Build history of the part. All positions in model axes, mm. Face numbers are marked on the shaded views. Coordinates: 2 decimals unless noted, no trailing zeros. Write each loop counter-clockwise with the first axis right and the second up, starting at its lowest first coordinate (ties: lowest second). Pieces come first, ordered by that corner, then holes.
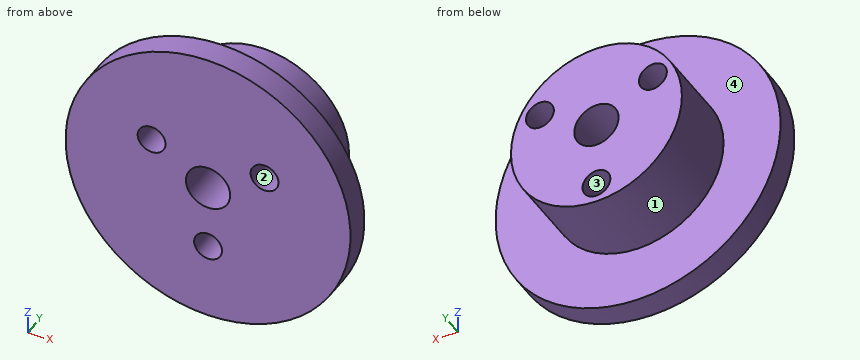
```python
from build123d import *

# Parameters (mm, degrees)
SKETCH_1_R          = 11.25
EXTRUDE_1_DEPTH     = 8
CUT_EXTRUDE_START   = -6
SKETCH_3_R          = 11.25
SKETCH_3_R_2        = 6.75
CUT_EXTRUDE_1_DEPTH = 6
SKETCH_4_R          = 1.75
SKETCH_4_R_2        = 1.1
CUT_EXTRUDE_2_DEPTH = 18.808003819


with BuildPart() as part:
    # 草图1 → 凸台-拉伸1 (new body)
    with BuildSketch(Plane(origin=(0, 0, 0), x_dir=(1, 0, 0), z_dir=(0, 1, 0))):
        with Locations(Location((0, 0, 0), (0, 0, 270))):
            Circle(SKETCH_1_R)
    extrude(amount=EXTRUDE_1_DEPTH)

    # 草图3 → 切除-拉伸1 (cut)
    with BuildSketch(Plane(origin=(0, 8, 0), x_dir=(1, 0, 0), z_dir=(0, 1, 0)).offset(CUT_EXTRUDE_START)):
        with Locations(Location((0, 0, 0), (0, 0, 270))):
            Circle(SKETCH_3_R)
        with Locations(Location((0, 0, 0), (0, 0, 270))):
            Circle(SKETCH_3_R_2, mode=Mode.SUBTRACT)
    extrude(amount=CUT_EXTRUDE_1_DEPTH, mode=Mode.SUBTRACT)

    # 草图4 → 切除-拉伸2 (cut, through all)
    with BuildSketch(Plane(origin=(0, 8, 0), x_dir=(1, 0, 0), z_dir=(0, 1, 0))):
        with Locations(Location((0, 0, 0), (0, 0, 270))):
            Circle(SKETCH_4_R)
        with Locations(Location((0, 5.15, 0), (0, 0, 270))):
            Circle(SKETCH_4_R_2)
        with Locations(Location((4.460030829, -2.575, 0), (0, 0, 270))):
            Circle(SKETCH_4_R_2)
        with Locations(Location((-4.460030829, -2.575, 0), (0, 0, 270))):
            Circle(SKETCH_4_R_2)
    extrude(amount=-CUT_EXTRUDE_2_DEPTH, mode=Mode.SUBTRACT)


solid = part.part
```
1. Saw through at D-D on y = 6.5. List the corners of the cut face in (x, z) (3 decimals).
Computed values:
outline: circle Ø13.5 at (0, 0); hole circle Ø2.2 at (-4.46, 2.575); hole circle Ø3.5 at (0, 0); hole circle Ø2.2 at (0, -5.15); hole circle Ø2.2 at (4.46, 2.575)
2. Flat gauge pins, fed straight in: pin 1 (4 mm diameter, centred on y = 2, z = -7.5, fed in from -X); pin 2 (1.5 mm diameter, centred on y = 2.5, z = -8, fed in from -X); pin 3 (1 mm diameter, centred on y = 5, z = 4, fed in from +X). Where does each tip first touch, or does it go through?
Computed values:
pin 1: stops at x = -9.81
pin 2: stops at x = -8.44
pin 3: stops at x = 5.77
3. Saw through at B-B on z = 0. List the corners of the cut face in (x, y), plus the area to 3 significant figures.
Computed values:
outline: (-11.25, 0) - (-1.75, 0) - (-1.75, 8) - (-6.75, 8) - (-6.75, 2) - (-11.25, 2) - close; (1.75, 0) - (11.25, 0) - (11.25, 2) - (6.75, 2) - (6.75, 8) - (1.75, 8) - close
area: 98.0 mm2
4. Probe line 1 along X through (y, z) = (6, 0); line 2 along X through (y, z) = (3, 3); line 3 along Y through (x, z) = (1.75, 7.5). List the from-to ranges inside material, lowest first.
Computed values:
line 1: x = -6.75 to -1.75, 1.75 to 6.75
line 2: x = -6.05 to -5.47, -3.45 to 3.45, 5.47 to 6.05
line 3: y = 0 to 2
5. Mould opens along Z. For the marked faces 1, 2, 3 and 4 say: +Z half, -Z half, draft (parallel to the pull), parting line (faces both ways), or undercut.
Computed values:
face 1: parting line
face 2: undercut
face 3: undercut
face 4: draft
6. Saw through at A-A on x = 0. List the corners of the cut face in (y, z), plus the area to 3 significant figures.
Computed values:
outline: (0, -11.25) - (2, -11.25) - (2, -6.75) - (8, -6.75) - (8, -6.25) - (0, -6.25) - close; (0, -4.05) - (8, -4.05) - (8, -1.75) - (0, -1.75) - close; (0, 1.75) - (8, 1.75) - (8, 6.75) - (2, 6.75) - (2, 11.25) - (0, 11.25) - close
area: 80.4 mm2
7. Saw through at C-C on x = 3.75. List the corners of the cut face in (y, z), plus the area to 3 significant figures.
Computed values:
outline: (0, -10.61) - (2, -10.61) - (2, -5.61) - (8, -5.61) - (8, 1.73) - (0, 1.73) - close; (0, 3.42) - (8, 3.42) - (8, 5.61) - (2, 5.61) - (2, 10.61) - (0, 10.61) - close
area: 96.3 mm2
